from build123d import *

# Parameters (mm, degrees)
SKETCH2_W           = 130
SKETCH2_H           = 90
BOSS_EXTRUDE1_DEPTH = 10
SKETCH3_W           = 42
SKETCH3_H           = 72
BOSS_EXTRUDE3_DEPTH = 53
SKETCH4_W           = 32
SKETCH4_H           = 43
CUT_EXTRUDE1_DEPTH  = 72
SKETCH5_R           = 6
CUT_EXTRUDE2_DEPTH  = 10
SKETCH6_W           = 72
SKETCH6_H           = 5
BOSS_EXTRUDE4_DEPTH = 48
SKETCH7_R           = 7.55
SKETCH7_R_2         = 1.6
CUT_EXTRUDE3_DEPTH  = 5
SKETCH8_R           = 6
CUT_EXTRUDE4_DEPTH  = 10
MIRROR2_OUTLINE_R   = 6
MIRROR2_DEPTH       = 10
SKETCH9_W           = 68
SKETCH9_H           = 43.95
BOSS_EXTRUDE5_DEPTH = 9
SKETCH10_W          = 7
SKETCH10_H          = 36
CUT_EXTRUDE5_DEPTH  = 5
BOSS_EXTRUDE6_DEPTH = 9
BOSS_EXTRUDE7_DEPTH = 9
SKETCH13_W          = 90
SKETCH13_H          = 63
BOSS_EXTRUDE8_DEPTH = 10


# Read off the part's stored shape, not the designer's step: Mirror2
with BuildPart() as part:
    # Sketch2 → Boss-Extrude1 (new body)
    with BuildSketch(Plane(origin=(0, 0, 0), x_dir=(1, 0, 0), z_dir=(0, 1, 0))):
        with Locations((0, 45)):
            Rectangle(SKETCH2_W, SKETCH2_H)
    extrude(amount=BOSS_EXTRUDE1_DEPTH)

    # Sketch3 → Boss-Extrude3 (add)
    with BuildSketch(Plane(origin=(0, 10, 0), x_dir=(1, 0, 0), z_dir=(0, 1, 0))):
        with Locations((45, 45)):
            Rectangle(SKETCH3_W, SKETCH3_H)
    boss_extrude3 = extrude(amount=BOSS_EXTRUDE3_DEPTH)

    # Sketch4 → Cut-Extrude1 (cut)
    with BuildSketch(Plane.XY.offset(-9)):
        with Locations((50, 31.5)):
            Rectangle(SKETCH4_W, SKETCH4_H)
    cut_extrude1 = extrude(amount=-CUT_EXTRUDE1_DEPTH, mode=Mode.SUBTRACT)

    # Sketch5 → Cut-Extrude2 (cut)
    with BuildSketch(Plane(origin=(0, 63, 0), x_dir=(1, 0, 0), z_dir=(0, 1, 0))):
        with Locations(Location((45, 45, 0), (0, 0, 270))):
            Circle(SKETCH5_R)
    cut_extrude2 = extrude(amount=-CUT_EXTRUDE2_DEPTH, mode=Mode.SUBTRACT)

    # Mirror1: Boss-Extrude3, Cut-Extrude1, Cut-Extrude2 across Right Plane
    add(boss_extrude3.mirror(Plane(origin=(0, 0, 0), x_dir=(0, 0, -1), z_dir=(1, 0, 0))))
    add(cut_extrude1.mirror(Plane(origin=(0, 0, 0), x_dir=(0, 0, -1), z_dir=(1, 0, 0))), mode=Mode.SUBTRACT)
    add(cut_extrude2.mirror(Plane(origin=(0, 0, 0), x_dir=(0, 0, -1), z_dir=(1, 0, 0))), mode=Mode.SUBTRACT)

    # Sketch6 → Boss-Extrude4 (add)
    with BuildSketch(Plane.ZY.offset(-24)):
        with Locations((-45, 51.45)):
            Rectangle(SKETCH6_W, SKETCH6_H)
    extrude(amount=BOSS_EXTRUDE4_DEPTH)

    # Sketch7 → Cut-Extrude3 (cut)
    with BuildSketch(Plane(origin=(0, 53.95, 0), x_dir=(1, 0, 0), z_dir=(0, 1, 0))):
        with Locations(Location((0, 45, 0), (0, 0, 270))):
            Circle(SKETCH7_R)
        with Locations(Location((12.005, 45, 0), (0, 0, 270))):
            Circle(SKETCH7_R_2)
        with Locations(Location((-12.005, 45, 0), (0, 0, 270))):
            Circle(SKETCH7_R_2)
    extrude(amount=-CUT_EXTRUDE3_DEPTH, mode=Mode.SUBTRACT)

    # Sketch8 → Cut-Extrude4 (cut)
    with BuildSketch(Plane(origin=(0, 10, 0), x_dir=(1, 0, 0), z_dir=(0, 1, 0))):
        with Locations(Location((49, 74, 0), (0, 0, 270))):
            Circle(SKETCH8_R)
    extrude(amount=-CUT_EXTRUDE4_DEPTH, mode=Mode.SUBTRACT)

    # Mirror2 outline → Mirror2 (cut)
    with BuildSketch(Plane(origin=(0, 0, 0), x_dir=(1, 0, 0), z_dir=(0, 1, 0))):
        with Locations((49, 16)):
            Circle(MIRROR2_OUTLINE_R)
        with Locations((-49, 74)):
            Circle(MIRROR2_OUTLINE_R)
        with Locations((-49, 16)):
            Circle(MIRROR2_OUTLINE_R)
    extrude(amount=MIRROR2_DEPTH, mode=Mode.SUBTRACT)

    # Sketch9 → Boss-Extrude5 (add)
    with BuildSketch(Plane.XY.offset(-9)):
        with Locations((0, 31.975)):
            Rectangle(SKETCH9_W, SKETCH9_H)
    extrude(amount=BOSS_EXTRUDE5_DEPTH)

    # Sketch10 → Cut-Extrude5 (cut)
    with BuildSketch(Plane(origin=(0, 53.95, 0), x_dir=(1, 0, 0), z_dir=(0, 1, 0))):
        with Locations((0, 63)):
            Rectangle(SKETCH10_W, SKETCH10_H)
    extrude(amount=-CUT_EXTRUDE5_DEPTH, mode=Mode.SUBTRACT)

    # Sketch11 → Boss-Extrude6 (add)
    with BuildSketch(Plane.XY.offset(-9)):
        Polygon((-66, 63), (-66, 53), (-34, 53), (-34, 53.95), (-24, 53.95), (-24, 63), align=None)
    boss_extrude6 = extrude(amount=BOSS_EXTRUDE6_DEPTH)

    # Mirror3: Boss-Extrude6 across Right Plane
    add(boss_extrude6.mirror(Plane(origin=(0, 0, 0), x_dir=(0, 0, -1), z_dir=(1, 0, 0))))

    # Sketch12 → Boss-Extrude7 (add)
    with BuildSketch(Plane(origin=(0, 0, -81), x_dir=(-1, 0, 0), z_dir=(0, 0, -1))):
        Polygon((-66, 63), (-66, 53), (-34, 53), (-34, 10), (-24, 10), (-24, 48.95), (-3.5, 48.95), (-3.5, 53.95), (-24, 53.95), (-24, 63), align=None)
    boss_extrude7 = extrude(amount=BOSS_EXTRUDE7_DEPTH)

    # Mirror4: Boss-Extrude7 across Right Plane
    add(boss_extrude7.mirror(Plane(origin=(0, 0, 0), x_dir=(0, 0, -1), z_dir=(1, 0, 0))))

    # Sketch13 → Boss-Extrude8 (add)
    with BuildSketch(Plane.ZY.offset(65)):
        with Locations((-45, 31.5)):
            Rectangle(SKETCH13_W, SKETCH13_H)
    boss_extrude8 = extrude(amount=BOSS_EXTRUDE8_DEPTH)

    # Mirror5: Boss-Extrude8 across Right Plane
    add(boss_extrude8.mirror(Plane(origin=(0, 0, 0), x_dir=(0, 0, -1), z_dir=(1, 0, 0))))


solid = part.part
Input: part model. Units: mm. Frame: model coordinates. A direction names the side the tool comes from. Coordinates: 2 decimals unless noted, no trailing zeros. Order: outer loops, then holes, each group sorted by start corner. A loop starts at its lowest first (then second) coordinate and runs counter-clockwise, first axis right, second up. Notation, with made-up numbers: M -16.5,-27.75 L 29.5,-27.75 A16 ccw 29.5,-0.75 Z; hole C 22.5,-22.5 d11. An arc over 180 degrees is marked long. Answer in a Markdown table with one row per item.
(1) Section query A-A, the plane z = -33.5. Output: boundary loops of the cut face in (x, y).
Numbers:
| item | result |
|---|---|
| outline | M -75,0 L 75,0 L 75,63 L 24,63 L 24,53.95 L -24,53.95 L -24,63 L -75,63 Z; hole M -65,10 L -34,10 L -34,53 L -65,53 Z; hole M -24,10 L 24,10 L 24,48.95 L -24,48.95 Z; hole M 34,10 L 65,10 L 65,53 L 34,53 Z |
(2) Section query D-D, the plane y = 6. Output: boundary loops of the cut face in (x, z).
Numbers:
| item | result |
|---|---|
| outline | M -75,-90 L 75,-90 L 75,0 L -75,0 Z; hole C -49,-74 d12; hole C -49,-16 d12; hole C 49,-74 d12; hole C 49,-16 d12 |
(3) Section query B-B, the plane y = 36.5. Output: boundary loops of the cut face in (x, z), plus the area to 3 significant figures.
Numbers:
| item | result |
|---|---|
| outline | M -75,-90 L -65,-90 L -65,0 L -75,0 Z; M -34,-90 L -24,-90 L -24,-9 L 24,-9 L 24,-90 L 34,-90 L 34,0 L -34,0 Z; M 65,-90 L 75,-90 L 75,0 L 65,0 Z |
| area | 4,030 mm^2 |
(4) Contact query for flat-ended pins moving along their axis: pin 1 Ø14.5 at (x, z) = (-9, -42) entering from +Y; pin 2 Ø9.5 at (x, z) = (45, -45) entering from +Y; pin 3 Ø11 at (x, z) = (-49, -74) entering from -Y. Output: stop coordinate, or through.
Numbers:
| item | result |
|---|---|
| pin 1 | stops at y = 53.95 |
| pin 2 | stops at y = 10 |
| pin 3 | stops at y = 53 |
(5) Draft query along X for faces 1 (the flat face through (-1, 31, 0)), 2 (the flat face through (49, 10, -46)), 3 (the cylindrical face through (-0.281, 51.485, -37.455)), 4 (the flat face through (-75, 32, -46)). Return one class per face: pulls with the +X half, pulls with the -X half, needs draft (parallel to the pull), parting line crosses it, or undercut.
Numbers:
| item | result |
|---|---|
| face 1 | needs draft |
| face 2 | undercut |
| face 3 | undercut |
| face 4 | pulls with the -X half |
(6) Material intervals for line 1 (X direction, y = 22, z = -31); line 2 (X direction, y = 59, z = -45); line 3 (Z direction, x = -49, y = 7.5), sorted ascending. Write a range as [from, to].
Numbers:
| item | result |
|---|---|
| line 1 | x = [-75, -65], [-34, -24], [24, 34], [65, 75] |
| line 2 | x = [-75, -51], [-39, -24], [24, 39], [51, 75] |
| line 3 | z = [-90, -80], [-68, -22], [-10, 0] |
(7) Section query C-C, the plane z = -5.5. Output: boundary loops of the cut face in (x, y), plus the area to 3 significant figures.
Numbers:
| item | result |
|---|---|
| outline | M -75,0 L 75,0 L 75,63 L 24,63 L 24,53.95 L -24,53.95 L -24,63 L -75,63 Z; hole M -65,10 L -34,10 L -34,53 L -65,53 Z; hole M 34,10 L 65,10 L 65,53 L 34,53 Z |
| area | 6,350 mm^2 |
(8) Access query for faces 5 (the cylindrical face through (45, 58, -51)), 6 (the flat face through (53, 53, -44)), 7 (the flat face through (24, 58, -44)). Directions: +Z, -Z, +X, -X, +Y, -Y. A direction counts if a zero-diameter tool reaches every point of the face in a straight line with its end or side. Return the directions, or none.
Numbers:
| item | result |
|---|---|
| face 5 | +Y |
| face 6 | +Z, -Z |
| face 7 | +Z, -Z, +Y |
